Geometry: final body of the model. Coordinates: model frame, mm. Face numbers are marked on the shaded views. Coordinates: 2 decimals unless noted, no trailing zeros. Write each loop counter-clockwise with the first axis right and the second up, starting at its lowest first coordinate (ties: lowest second). Pieces come first, ordered by that corner, then holes.
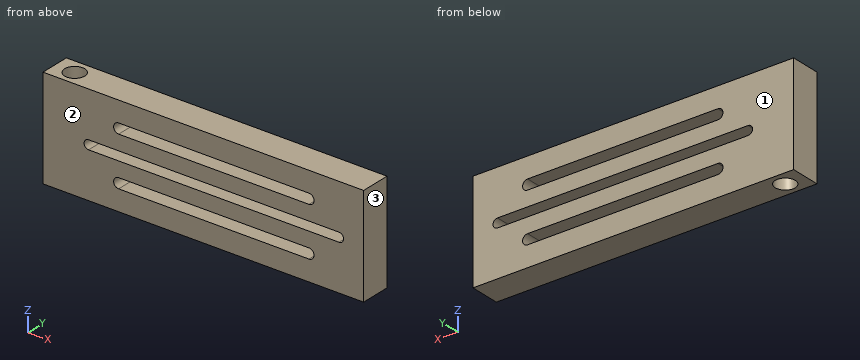
from build123d import *

# Parameters (mm, degrees)
SKETCH1_W           = 203.2
SKETCH1_H           = 63.5
BOSS_EXTRUDE1_DEPTH = 9.525
CUT_EXTRUDE1_DEPTH  = 109.136603424
CUT_EXTRUDE2_REACH  = 122.19
SKETCH3_R           = 6.35


with BuildPart() as part:
    # Sketch1 → Boss-Extrude1 (new, symmetric)
    with BuildSketch(Plane(origin=(0, 0, 0), x_dir=(1, 0, 0), z_dir=(0, 1, 0))):
        Rectangle(SKETCH1_W, SKETCH1_H)
    extrude(amount=BOSS_EXTRUDE1_DEPTH, both=True)

    # Sketch2 → Cut-Extrude1 (cut, through all)
    with BuildSketch(Plane(origin=(0, 9.525, 0), x_dir=(1, 0, 0), z_dir=(0, 1, 0))):
        with BuildLine():
            Line((-72.7075, 2.8575), (86.0425, 2.8575))
            ThreePointArc((86.0425, 2.8575), (88.9, 0), (86.0425, -2.8575))
            Line((86.0425, -2.8575), (-72.7075, -2.8575))
            ThreePointArc((-72.7075, -2.8575), (-75.565, 0), (-72.7075, 2.8575))
        make_face()
        with BuildLine():
            Line((-53.6575, 18.7325), (66.9925, 18.7325))
            ThreePointArc((66.9925, 18.7325), (70.1675, 15.5575), (66.9925, 12.3825))
            Line((66.9925, 12.3825), (-53.6575, 12.3825))
            ThreePointArc((-53.6575, 12.3825), (-56.8325, 15.5575), (-53.6575, 18.7325))
        make_face()
        with BuildLine():
            Line((-53.6575, -12.3825), (66.9925, -12.3825))
            ThreePointArc((66.9925, -12.3825), (70.1675, -15.5575), (66.9925, -18.7325))
            Line((66.9925, -18.7325), (-53.6575, -18.7325))
            ThreePointArc((-53.6575, -18.7325), (-56.8325, -15.5575), (-53.6575, -12.3825))
        make_face()
    extrude(amount=-CUT_EXTRUDE1_DEPTH, mode=Mode.SUBTRACT)

    # Sketch3 → Cut-Extrude2 (cut, up to next)
    with BuildSketch(Plane(origin=(0, 0, -31.75), x_dir=(-1, 0, 0), z_dir=(0, 0, -1)), mode=Mode.PRIVATE) as cut_extrude2_sk1:
        with Locations((88.9, 0)):
            Circle(SKETCH3_R)
    cut_extrude2_tool1 = extrude(cut_extrude2_sk1.sketch, amount=-CUT_EXTRUDE2_REACH, mode=Mode.PRIVATE) & part.part
    add(cut_extrude2_tool1.solids().sort_by_distance((-88.9, 0, -31.75))[0], mode=Mode.SUBTRACT)


solid = part.part
Item 1: Pin query (flat end, axial travel): pin 1 (12 mm diameter, centred on x = -13, z = -15, fed in from +Y) (3 decimals). Return the tip coordinate at first contact, or that it passes through.
Derived:
pin 1: stops at y = 9.525
Item 2: Section B-B, the plane z = 0. Output: boundary loops of the cut face in (x, y) (3 decimals).
Derived:
outline: (-101.6, -9.525) - (-75.565, -9.525) - (-75.565, 9.525) - (-101.6, 9.525) - close; (88.9, -9.525) - (101.6, -9.525) - (101.6, 9.525) - (88.9, 9.525) - close; hole circle Ø12.7 at (-88.9, 0)
Item 3: Material intervals for probe 1 along Z at (x, y) = (4, 3.75); probe 2 along Y at (x, z) = (-88.9, -8.5) (3 decimals); probe 3 along Z at (x, y) = (77.5, 2.5), sorted ascending.
Derived:
probe 1: z = -31.75 to -18.73, -12.38 to -2.86, 2.86 to 12.38, 18.73 to 31.75
probe 2: y = -9.525 to -6.35, 6.35 to 9.525
probe 3: z = -31.75 to -2.86, 2.86 to 31.75
Item 4: Pull-direction query (Y, two-part tool) for the marked faces 1, 2 and 3; classes: released by +Y, released by -Y, zero draft, split by the parting line, or undercut.
Derived:
face 1: released by +Y
face 2: released by -Y
face 3: zero draft
Item 5: Section A-A, the plane y = 0. State how many separate pieces and enclosed holes the cut face has, plus the area to 3 significant figures.
Derived:
separate pieces: 2
enclosed holes: 3
area: 9,570 mm2
Item 6: Section C-C, the plane x = -88.9. Output: boundary loops of the cut face in (y, z) (3 decimals), plus the area to 3 significant figures.
Derived:
outline: (-9.525, -31.75) - (-6.35, -31.75) - (-6.35, 31.75) - (-9.525, 31.75) - close; (6.35, -31.75) - (9.525, -31.75) - (9.525, 31.75) - (6.35, 31.75) - close
area: 403 mm2
